```python
from build123d import *

# Parameters (mm, degrees)
F0_R     = 11.2
F1_DEPTH = 7


with BuildPart() as f1:
    # F0 (on Top) → F1 (new body)
    with BuildSketch(Plane.XY):
        with BuildLine():
            ThreePointArc((-13.18295, 27.738768), (-20.872941, 20.982416), (-26.569568, 12.477552))
            ThreePointArc((-26.569568, 12.477552), (-49.879326, 0.682754), (-27.738768, -13.18295))
            ThreePointArc((-27.738768, -13.18295), (-20.982416, -20.872941), (-12.477552, -26.569568))
            ThreePointArc((-12.477552, -26.569568), (-0.682754, -49.879326), (13.18295, -27.738768))
            ThreePointArc((13.18295, -27.738768), (20.872941, -20.982416), (26.569568, -12.477552))
            ThreePointArc((26.569568, -12.477552), (49.879326, -0.682754), (27.738768, 13.18295))
            ThreePointArc((27.738768, 13.18295), (20.982416, 20.872941), (12.477552, 26.569568))
            ThreePointArc((12.477552, 26.569568), (0.682754, 49.879326), (-13.18295, 27.738768))
        make_face()
        with BuildLine():
            Line((-20.646999, 15.66407), (-11.071281, 7.187957))
            ThreePointArc((-11.071281, 7.187957), (-13.160123, -1.025268), (-9.824467, -8.815886))
            Line((-9.824467, -8.815886), (-18.350719, -18.448246))
            ThreePointArc((-18.350719, -18.448246), (-21.599994, -14.678222), (-24.015539, -10.32667))
            ThreePointArc((-24.015539, -10.32667), (-19.897377, -0.274085), (-23.645482, 9.922259))
            ThreePointArc((-23.645482, 9.922259), (-22.337874, 12.893239), (-20.646999, 15.66407))
        make_face(mode=Mode.SUBTRACT)
        with Locations((0, -34.894872)):
            Circle(F0_R, mode=Mode.SUBTRACT)
        with BuildLine():
            ThreePointArc((10.32667, -24.015539), (0.274085, -19.897377), (-9.922259, -23.645482))
            ThreePointArc((-9.922259, -23.645482), (-12.893239, -22.337874), (-15.66407, -20.646999))
            Line((-15.66407, -20.646999), (-7.187957, -11.071281))
            ThreePointArc((-7.187957, -11.071281), (1.025268, -13.160123), (8.815886, -9.824467))
            Line((8.815886, -9.824467), (18.448246, -18.350719))
            ThreePointArc((18.448246, -18.350719), (14.678222, -21.599994), (10.32667, -24.015539))
        make_face(mode=Mode.SUBTRACT)
        with Locations((-34.894872, 0)):
            Circle(F0_R, mode=Mode.SUBTRACT)
        with BuildLine():
            ThreePointArc((-18.448246, 18.350719), (-14.678222, 21.599994), (-10.32667, 24.015539))
            ThreePointArc((-10.32667, 24.015539), (-0.274085, 19.897377), (9.922259, 23.645482))
            ThreePointArc((9.922259, 23.645482), (12.893239, 22.337874), (15.66407, 20.646999))
            Line((15.66407, 20.646999), (7.187957, 11.071281))
            ThreePointArc((7.187957, 11.071281), (-1.025268, 13.160123), (-8.815886, 9.824467))
            Line((-8.815886, 9.824467), (-18.448246, 18.350719))
        make_face(mode=Mode.SUBTRACT)
        Circle(F0_R, mode=Mode.SUBTRACT)
        with BuildLine():
            ThreePointArc((18.350719, 18.448246), (21.599994, 14.678222), (24.015539, 10.32667))
            ThreePointArc((24.015539, 10.32667), (19.897377, 0.274085), (23.645482, -9.922259))
            ThreePointArc((23.645482, -9.922259), (22.337874, -12.893239), (20.646999, -15.66407))
            Line((20.646999, -15.66407), (11.071281, -7.187957))
            ThreePointArc((11.071281, -7.187957), (13.160123, 1.025268), (9.824467, 8.815886))
            Line((9.824467, 8.815886), (18.350719, 18.448246))
        make_face(mode=Mode.SUBTRACT)
        with Locations((34.894872, 0)):
            Circle(F0_R, mode=Mode.SUBTRACT)
        with Locations((0, 34.894872)):
            Circle(F0_R, mode=Mode.SUBTRACT)
    extrude(amount=F1_DEPTH)


solid = f1.part
```
Could you check a few things on this model? Use its own coordinates, in mm. A direction names the side the tool comes from. Round coordinates to 2 decimals unless told otherwise and drop trailing zeros. Loops run counter-clockwise (first coordinate to the right, second up) from the corner with the lowest first, then second, coordinate; pieces in that order, holes last. Notation, with made-up numbers: (40.5, 13) -> (71.5, 13) arc R19 cw to (71.5, 21) -> close; hole circle Ø11 at (-34, 15). An arc over 180 degrees is marked (long way). One line per question, with ' | ' between items.
(1) If we section it at D-D on y = -41: List the corners of the cut face in (x, z) for me, and give its area (3 significant figures).
Model answer:
outline: (-13.7, 0) -> (-9.39, 0) -> (-9.39, 7) -> (-13.7, 7) -> close; (9.39, 0) -> (13.7, 0) -> (13.7, 7) -> (9.39, 7) -> close | area: 60.4 mm^2
(2) For faces 1 (the face through (-4, -11, 0)), 2 (the face through (-11.49, -15.93, 3.45)), which set-ups out of +Z, -Z, +X, -X, +Y, -Y let a thin tool reach every point of the face, with its end or its side?
Model answer:
face 1: -Z, +X, -X, +Y, -Y | face 2: +Z, -Z
(3) For pin 1 Ø1.5 at (y, z) = (25, 3.5) entering from +X; pin 2 Ø2 at (x, z) = (-37, 3) entering from -Y; pin 3 Ø2 at (x, z) = (24.5, 2) entering from -Y, each with a flat end and sliding along its axis, tell me the tip position at first contact or that it passes through.
Model answer:
pin 1: stops at x = 16.53 | pin 2: stops at y = -14.96 | pin 3: stops at y = -17.64
(4) If we section it at C-C on x = 22.5: List the corners of the cut face in (y, z) for me, and give its area (3 significant figures).
Model answer:
outline: (-19, 0) -> (-12.58, 0) -> (-12.58, 7) -> (-19, 7) -> close; (-8.45, 0) -> (8.45, 0) -> (8.45, 7) -> (-8.45, 7) -> close; (13.29, 0) -> (19.47, 0) -> (19.47, 7) -> (13.29, 7) -> close | area: 207 mm^2
(5) If we section it at A-A on y = 0: List the corners of the cut face in (x, z) for me.
Model answer:
outline: (-49.89, 0) -> (-46.09, 0) -> (-46.09, 7) -> (-49.89, 7) -> close; (-23.69, 0) -> (-19.89, 0) -> (-19.89, 7) -> (-23.69, 7) -> close; (-13.2, 0) -> (-11.2, 0) -> (-11.2, 7) -> (-13.2, 7) -> close; (11.2, 0) -> (13.2, 0) -> (13.2, 7) -> (11.2, 7) -> close; (19.89, 0) -> (23.69, 0) -> (23.69, 7) -> (19.89, 7) -> close; (46.09, 0) -> (49.89, 0) -> (49.89, 7) -> (46.09, 7) -> close
(6) If I drill on probe 1 along Y at (x, z) = (0, 4.5); probe 2 along X at (y, z) = (-21, 2.25); probe 3 along Y at (x, z) = (-4, 2.5), over which ranges is the centre line in solid material (lowest first)?
Model answer:
probe 1: y = -49.89 to -46.09, -23.69 to -19.89, -13.2 to -11.2, 11.2 to 13.2, 19.89 to 23.69, 46.09 to 49.89 | probe 2: x = -20.84 to -15.15, -5.65 to 5.65, 15.5 to 20.86 | probe 3: y = -49.35 to -45.36, -24.43 to -20.44, -12.58 to -10.46, 10.46 to 12.58, 20.44 to 24.43, 45.36 to 49.35
